from build123d import *
from OCP.BRepFilletAPI import BRepFilletAPI_MakeChamfer

# Parameters (mm, degrees)
SKETCH1_R           = 0.625
BOSS_EXTRUDE1_DEPTH = 7.5
SKETCH2_R           = 1.325
BOSS_EXTRUDE2_DEPTH = 0.75
SKETCH3_W           = 0.3
SKETCH3_H           = 7.682003158
CUT_EXTRUDE1_DEPTH  = 0.15
CHAMFER1_SIZE       = 0.05
CHAMFER1_SIZE2      = 0.045176141
FILLET1_R           = 0.05
CHAMFER2_SIZE       = 0.05


with BuildPart() as part:
    # Sketch1 → Boss-Extrude1 (new body)
    with BuildSketch(Plane.XY):
        Circle(SKETCH1_R)
    extrude(amount=BOSS_EXTRUDE1_DEPTH)

    # Sketch2 → Boss-Extrude2 (add)
    with BuildSketch(Plane.XY):
        Circle(SKETCH2_R)
    extrude(amount=-BOSS_EXTRUDE2_DEPTH)

    # Sketch3 → Cut-Extrude1 (cut)
    with BuildSketch(Plane(origin=(0, 0, -0.75), x_dir=(-1, 0, 0), z_dir=(0, 0, -1))):
        Rectangle(SKETCH3_W, SKETCH3_H)
    extrude(amount=-CUT_EXTRUDE1_DEPTH, mode=Mode.SUBTRACT)

    # Chamfer1: one chamfer whose edges measure the first distance from different faces: ONE call of the kernel's chamfer builder (chamfer() names one face for all edges)
    chamfer1_edges_1 = [part.edges().sort_by_distance(p)[0] for p in [
        (-1.325, 0, -0.75),
        (0.988527946, 0.882291052, -0.75),
        (-0.15, 0, -0.75),
        (0.15, 0, -0.75),
        (0, 1.325, -0.6),
        (0, -1.325, -0.6),
        (0.15, 0, -0.6),
        (-0.15, 0, -0.6),
    ]]
    chamfer1_edges_2 = [part.edges().sort_by_distance(p)[0] for p in [
        (0.15, 1.316482055, -0.675),
        (0.15, -1.316482055, -0.675),
        (-0.15, -1.316482055, -0.675),
        (-0.15, 1.316482055, -0.675),
    ]]
    chamfer1_side_2 = [part.faces().sort_by_distance(p)[0] for p in [
        (-1.325, 0, -0.375),
    ]]
    chamfer1 = BRepFilletAPI_MakeChamfer(part.part.solid().wrapped)
    for e in chamfer1_edges_1:
        chamfer1.Add(CHAMFER1_SIZE, e.wrapped)
    for e in chamfer1_edges_2:
        chamfer1.Add(CHAMFER1_SIZE, CHAMFER1_SIZE2, e.wrapped, chamfer1_side_2[0].wrapped)  # the first distance lies on this face
    add(Compound.cast(chamfer1.Shape()), mode=Mode.REPLACE)

    # Fillet1
    fillet1_edges = [part.edges().sort_by_distance(p)[0] for p in [
        (-0.625, 0, 0),
        (-1.325, 0, 0),
    ]]
    fillet(fillet1_edges, radius=FILLET1_R)

    # Chamfer2
    chamfer2_edges = [part.edges().sort_by_distance(p)[0] for p in [
        (-0.625, 0, 7.5),
    ]]
    chamfer(chamfer2_edges, length=CHAMFER2_SIZE)


solid = part.part
Build history of the part. All positions in model axes, mm. A direction names the side the tool comes from. Round coordinates to 2 decimals unless told otherwise and drop trailing zeros. Loops run counter-clockwise (first coordinate to the right, second up) from the corner with the lowest first, then second, coordinate; pieces in that order, holes last. Notation, with made-up numbers: (77, 52.5) -> (119, 52.5) arc R19 cw to (119, 78.5) -> close; hole circle Ø8 at (24, -2.5). An arc over 180 degrees is marked (long way). One line per item, written item: value. Start each with the question number.
Q1. 3-axis set-ups, long thin cutter, end or side, ignore diameter. For faces 1 (the face through (1, 0, -0.75)), 2 (the face through (0, -1, 0)): which of +Z, -Z, +X, -X, +Y, -Y reach the whole face in a straight line?
Q2. Probe line 1 along Z through (x, y) = (-0.6, 0.85); line 2 along Z through (x, y) = (0, -1); line 3 along X through (y, z) = (0.35, 3.75). List the from-to ranges inside material, lowest first.
Q3. Cut at C-C on z = 6. List the corners of the cut face in (x, y) (3 decimals).
Q4. Cut at A-A on x = 0. List the corners of the cut face in (y, z) (3 decimals).
Q5. Drop flat-ended pins along their axis: pin 1 Ø1 at (x, y) = (-0.5, -0.5) entering from +Z; pin 2 Ø1 at (x, z) = (0.5, 1) entering from -Y (3 decimals). Give the stop position or say it passes through.
Q6. Cut at B-B on y = 0. List the corners of the cut face in (x, z) (3 decimals), plus the area to 3 significant figures.
Computed:
1. face 1: -Z, +X, -X, +Y, -Y
1. face 2: +Z
2. line 1: -0.75 to 0
2. line 2: -0.6 to 0
2. line 3: -0.52 to 0.52
3. outline: circle Ø1.25 at (0, 0)
4. outline: (-1.325, -0.55) -> (-1.275, -0.6) -> (1.275, -0.6) -> (1.325, -0.55) -> (1.325, -0.05) arc R0.05 ccw to (1.275, 0) -> (0.675, 0) arc R0.05 cw to (0.625, 0.05) -> (0.625, 7.45) -> (0.575, 7.5) -> (-0.575, 7.5) -> (-0.625, 7.45) -> (-0.625, 0.05) arc R0.05 cw to (-0.675, 0) -> (-1.275, 0) arc R0.05 ccw to (-1.325, -0.05) -> close
5. pin 1: z = 7.5
5. pin 2: y = -0.625
6. outline: (-1.325, -0.7) -> (-1.275, -0.75) -> (-0.2, -0.75) -> (-0.15, -0.7) -> (-0.15, -0.65) -> (-0.1, -0.6) -> (0.1, -0.6) -> (0.15, -0.65) -> (0.15, -0.7) -> (0.2, -0.75) -> (1.275, -0.75) -> (1.325, -0.7) -> (1.325, -0.05) arc R0.05 ccw to (1.275, 0) -> (0.675, 0) arc R0.05 cw to (0.625, 0.05) -> (0.625, 7.45) -> (0.575, 7.5) -> (-0.575, 7.5) -> (-0.625, 7.45) -> (-0.625, 0.05) arc R0.05 cw to (-0.675, 0) -> (-1.275, 0) arc R0.05 ccw to (-1.325, -0.05) -> close
6. area: 11.3 mm²
